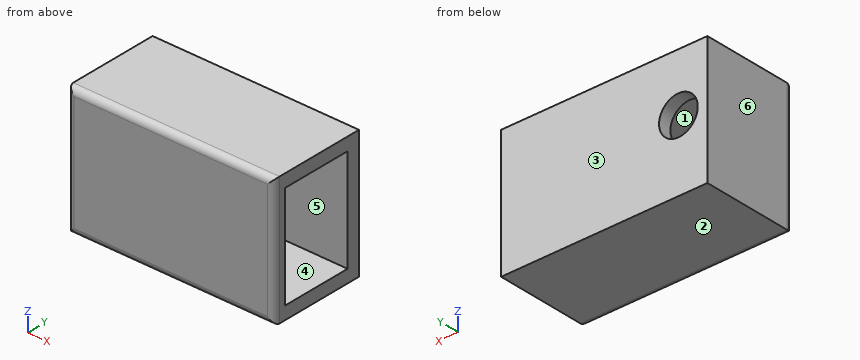
```python
from build123d import *

# Parameters (mm, degrees)
SKETCH1_W           = 30
SKETCH1_H           = 16
BOSS_EXTRUDE1_DEPTH = 11
SHELL1_T            = 2
CUT_EXTRUDE3_REACH  = 26.779
SKETCH4_R           = 3
FILLET1_R           = 1


with BuildPart() as part:
    # Sketch1 → Boss-Extrude1 (new body)
    with BuildSketch(Plane(origin=(0, 0, 0), x_dir=(1, 0, 0), z_dir=(0, 1, 0))):
        Rectangle(SKETCH1_W, SKETCH1_H)
    extrude(amount=BOSS_EXTRUDE1_DEPTH)

    # Shell1
    shell1_openings = [part.faces().sort_by_distance(p)[0] for p in [
        (15, 5.5, 0),
    ]]
    offset(amount=SHELL1_T, openings=shell1_openings, kind=Kind.INTERSECTION)

    # Cut-Extrude3: up to this face of the body (flat: up to its plane)
    cut_extrude3_end = Plane(part.part.faces().sort_by_distance((0, 0, 0))[0])
    # Sketch4 → Cut-Extrude3 (cut, up to the picked face)
    with BuildSketch(Plane(origin=(0, 13, 0), x_dir=(1, 0, 0), z_dir=(0, 1, 0)), mode=Mode.PRIVATE) as cut_extrude3_sk1:
        with Locations(Location((-12.5, -1, 0), (0, 0, 270))):
            Circle(SKETCH4_R)
    cut_extrude3_tool1 = split(extrude(cut_extrude3_sk1.sketch, amount=-CUT_EXTRUDE3_REACH, mode=Mode.PRIVATE), bisect_by=cut_extrude3_end, keep=Keep.BOTH, mode=Mode.PRIVATE)
    add(cut_extrude3_tool1.solids().sort_by(Axis((-12.5, 13, 1), (0, -1, 0)))[0], mode=Mode.SUBTRACT)

    # Fillet1
    fillet1_edges = [part.edges().sort_by_distance(p)[0] for p in [
        (-1, -2, 10),
        (-17, -2, 0),
        (-1, -2, -10),
        (15, -2, 0),
    ]]
    fillet(fillet1_edges, radius=FILLET1_R)


solid = part.part
```
CAD build for the part. Positions are in the model's coordinates, mm. Face numbers are marked on the shaded views. A direction names the side the tool comes from. Round coordinates to 2 decimals unless told otherwise and drop trailing zeros. Order: outer loops, then holes, each group sorted by start corner. A loop starts at its lowest first (then second) coordinate and runs counter-clockwise, first axis right, second up. Notation, with made-up numbers: (71, -10.75) -> (116, -10.75) arc R18 ccw to (116, 11.25) -> close; hole circle Ø11 at (47, -4.5). An arc over 180 degrees is marked (long way). Write item = value, one per line.
(1) Cut at C-C (y = 9). Write the cut outline in (x, z).
Answers follow:
outline = (-17, -10) -> (15, -10) -> (15, -8) -> (-15, -8) -> (-15, -0.66) arc R3 cw to (-15, 2.66) -> (-15, 8) -> (15, 8) -> (15, 10) -> (-17, 10) -> close
(2) Cut at D-D (x = -12.5). Write the cut outline in (y, z).
Answers follow:
outline = (-2, -9) arc R1 ccw to (-1, -10) -> (13, -10) -> (13, -2) -> (11, -2) -> (11, -8) -> (0, -8) -> (0, 8) -> (11, 8) -> (11, 4) -> (13, 4) -> (13, 10) -> (-1, 10) arc R1 ccw to (-2, 9) -> close
(3) Flat gauge pin, fed straight in: P1, Ø4.5, axis at y = 5.5, z = 5.5, coming from the +X side. Where does the tip first touch, or does it go through?
Answers follow:
P1 = -15
(4) Cut at A-A (z = 1). Write the cut outline in (x, y).
Answers follow:
outline = (-17, -1) arc R1 ccw to (-16, -2) -> (14, -2) arc R1 ccw to (15, -1) -> (15, 0) -> (-15.5, 0) -> (-15.5, 13) -> (-17, 13) -> close; (-9.5, 11) -> (15, 11) -> (15, 13) -> (-9.5, 13) -> close
(5) Drill centre lines: L1, parallel to Z at x = -3, y = 8.25; L2, parallel to Y at x = -7, z = -2.25; L3, parallel to X at y = 6.5, z = -2. Where is each one in solid material? Low to high.
Answers follow:
L1 = -10 to -8, 8 to 10
L2 = -2 to 0, 11 to 13
L3 = -17 to -15
(6) 3-axis set-ups, long thin cutter, end or side, ignore diameter. For the marked faces 5 and 6: which of +Z, -Z, +X, -X, +Y, -Y reach the whole face in a straight line?
Answers follow:
face_5 = +X
face_6 = +Z, -Z, -X, +Y, -Y
(7) Cut at B-B (x = -8.5). Write the cut outline in (y, z).
Answers follow:
outline = (-2, -9) arc R1 ccw to (-1, -10) -> (13, -10) -> (13, 10) -> (-1, 10) arc R1 ccw to (-2, 9) -> close; hole (0, -8) -> (11, -8) -> (11, 8) -> (0, 8) -> close
(8) Pull direction Z, two halves, no side cores. Call the marked faces 1, 2, 3 and 4: +Z half, -Z half, draft (parallel to the pull), parting line (faces both ways), or undercut.
Answers follow:
face_1 = undercut
face_2 = -Z half
face_3 = draft
face_4 = undercut
